from build123d import *

# Parameters (mm, degrees)
SKETCH1_W           = 25.4
SKETCH1_H           = 25.4
SKETCH1_W_2         = 22.225
SKETCH1_H_2         = 22.225
BOSS_EXTRUDE1_DEPTH = 711.2
SKETCH2_R           = 2.5527
CUT_EXTRUDE1_DEPTH  = 26.4
SKETCH3_R           = 2.5527
CUT_EXTRUDE2_DEPTH  = 26.4


with BuildPart() as part:
    # Sketch1 → Boss-Extrude1 (new body)
    with BuildSketch(Plane(origin=(0, 0, 0), x_dir=(1, 0, 0), z_dir=(0, 1, 0))):
        Rectangle(SKETCH1_W, SKETCH1_H)
        Rectangle(SKETCH1_W_2, SKETCH1_H_2, mode=Mode.SUBTRACT)
    extrude(amount=BOSS_EXTRUDE1_DEPTH)

    # Sketch2 → Cut-Extrude1 (cut, through all)
    with BuildSketch(Plane.XY.offset(12.7)):
        with Locations((0, 9.525)):
            Circle(SKETCH2_R)
        with Locations((0, 28.575)):
            Circle(SKETCH2_R)
        with Locations((0, 47.625)):
            Circle(SKETCH2_R)
    extrude(amount=-CUT_EXTRUDE1_DEPTH, mode=Mode.SUBTRACT)

    # Sketch3 → Cut-Extrude2 (cut, through all)
    with BuildSketch(Plane(origin=(12.7, 0, 0), x_dir=(0, 0, -1), z_dir=(1, 0, 0))):
        with Locations((0, 9.525)):
            Circle(SKETCH3_R)
        with Locations((0, 28.575)):
            Circle(SKETCH3_R)
        with Locations((0, 47.625)):
            Circle(SKETCH3_R)
        with Locations((0, 701.675)):
            Circle(SKETCH3_R)
        with Locations((0, 682.625)):
            Circle(SKETCH3_R)
    extrude(amount=-CUT_EXTRUDE2_DEPTH, mode=Mode.SUBTRACT)


solid = part.part
Can you work these out from the model? Positions are in its coordinate system, mm. A direction names the side the tool comes from. Round coordinates to 2 decimals unless told otherwise and drop trailing zeros. Write each loop counter-clockwise with the first axis right and the second up, starting at its lowest first coordinate (ties: lowest second). Pieces come first, ordered by that corner, then holes. Notation, with made-up numbers: (31.25, 32.5) -> (83.25, 32.5) arc R21 ccw to (83.25, 46.5) -> close; hole circle Ø11 at (48.5, -38). An arc over 180 degrees is marked (long way). Use one line per item in the form item = value. Start each with the question number.
Q1. If I drill on probe 1 along Y at (x, z) = (0, -11.85); probe 2 along Y at (x, z) = (11.75, 0); probe 3 along X at (y, z) = (140.5, 6), over which ranges is the centre line in solid material (lowest first)? Write a range as [from, to].
Q2. Imagine slicing it at A-A (y = 263.5). Please give me the cut outline in (x, z).
Q3. Which directions (+Z, -Z, +X, -X, +Y, -Y) give clear straight access to the entire face, cutting with the end or side of a thin tool? Please do faces 1 (the face through (0, 351, 12.7)), 2 (the face through (-11.112, 351, 0)).
Q4. We'd pull the mould along X, two halves only. Please class faces 3 (the face through (-12.7, 351, 0)), 4 (the face through (11.112, 351, 0)), 5 (the face through (-11.3, 0, -0.1)), 6 (the face through (0, 351, -11.112)): +X half, -X half, draft (parallel to the pull), parting line (faces both ways), or undercut.
Worked out:
q1.probe_1 = [0, 6.97], [12.08, 26.02], [31.13, 45.07], [50.18, 711.2]
q1.probe_2 = [0, 6.97], [12.08, 26.02], [31.13, 45.07], [50.18, 680.07], [685.18, 699.12], [704.23, 711.2]
q1.probe_3 = [-12.7, -11.11], [11.11, 12.7]
q2.outline = (-12.7, -12.7) -> (12.7, -12.7) -> (12.7, 12.7) -> (-12.7, 12.7) -> close; hole (-11.11, -11.11) -> (11.11, -11.11) -> (11.11, 11.11) -> (-11.11, 11.11) -> close
q3.face_1 = +Z, +X, -X, +Y, -Y
q3.face_2 = +Y, -Y
q4.face_3 = -X half
q4.face_4 = undercut
q4.face_5 = draft
q4.face_6 = undercut
